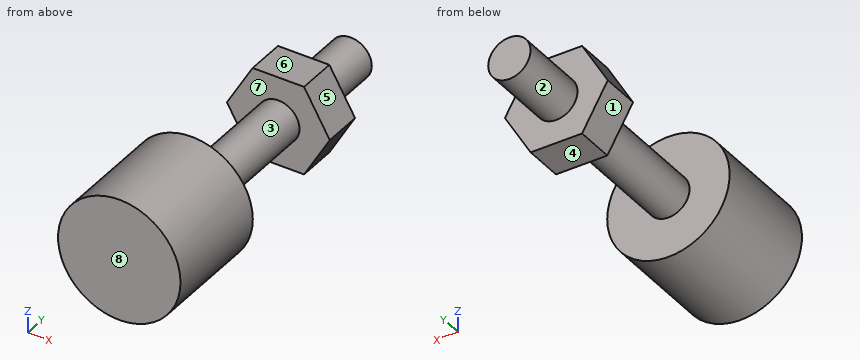
from build123d import *

# Parameters (mm, degrees)
F0_R     = 5.5
F0_R_2   = 1.9
F1_DEPTH = 10
F2_DEPTH = 22
F4_START = -6.5
F4_DEPTH = 3.5


with BuildPart() as f1:
    # F0 (on Front) → F1 (new body)
    with BuildSketch(Plane.XZ):
        Circle(F0_R)
        Circle(F0_R_2, mode=Mode.SUBTRACT)
        Circle(F0_R_2)
    extrude(amount=F1_DEPTH)

    # F0 (on Front) → F2 (join)
    with BuildSketch(Plane.XZ):
        Circle(F0_R_2)
    extrude(amount=-F2_DEPTH)

    # F3 (on face) → F4 (join)
    with BuildSketch(Plane(origin=(0, 22, 0), x_dir=(-1, 0, 0), z_dir=(0, 1, 0)).offset(F4_START)):
        Polygon((2.3094010768, 4), (-2.3094010768, 4), (-4.6188021535, 0), (-2.3094010768, -4), (2.3094010768, -4), (4.6188021535, 0), align=None)
    extrude(amount=-F4_DEPTH)


solid = f1.part
Build history of the part. All positions in model axes, mm. Face numbers are marked on the shaded views. A direction names the side the tool comes from. Give positions to 0.01 mm unless a question says otherwise; leave off trailing zeros. Order: outer loops, then holes, each group sorted by start corner. A loop starts at its lowest first (then second) coordinate and runs counter-clockwise, first axis right, second up. Notation, with made-up numbers: M 22.5,-35 L 57.5,-35 A29 cw 57.5,-6 Z; hole C 0.5,48 d8. An arc over 180 degrees is marked long. Use one line per item in the form item = value.
1) Saw through at C-C (y = -4). Give the cut face in (x, z), plus the area to 3 significant figures.
Calculated:
outline = C 0,0 d11
area = 95.0 mm2
2) Saw through at D-D (y = 16). Give the cut face in (x, z), plus the area to 3 significant figures.
Calculated:
outline = C 0,0 d3.8
area = 11.3 mm2
3) Saw through at A-A (x = 0). Give the cut face in (y, z), plus the area to 3 significant figures.
Calculated:
outline = M -10,-5.5 L 0,-5.5 L 0,-1.9 L 12,-1.9 L 12,-4 L 15.5,-4 L 15.5,-1.9 L 22,-1.9 L 22,1.9 L 15.5,1.9 L 15.5,4 L 12,4 L 12,1.9 L 0,1.9 L 0,5.5 L -10,5.5 Z
area = 208 mm2
4) Tool access for the marked faces 1, 2, 3, 4 and 5: list every direction of +Z, -Z, +X, -X, +Y, -Y with a clear straight run to the whole face (end or side of a thin tool).
Calculated:
face_1 = -Z, -X, +Y
face_2 = +Y
face_3 = none
face_4 = -Z, +X, -X, +Y
face_5 = +Z, +X, +Y
5) Saw through at B-B (z = 1). Give the cut face in (x, y).
Calculated:
outline = M -5.41,-10 L 5.41,-10 L 5.41,0 L 1.62,0 L 1.62,12 L 4.04,12 L 4.04,15.5 L 1.62,15.5 L 1.62,22 L -1.62,22 L -1.62,15.5 L -4.04,15.5 L -4.04,12 L -1.62,12 L -1.62,0 L -5.41,0 Z
6) Probe probe 1 along Y at (x, z) = (-3, -1.75); probe 2 along Y at (x, z) = (-5, -1.25); probe 3 along X at (y, z) = (16.5, -0.5). List the from-to ranges inside material, lowest first.
Calculated:
probe_1 = -10 to 0, 12 to 15.5
probe_2 = -10 to 0
probe_3 = -1.83 to 1.83
7) Two-plate mould, pull along Y, no slides. Class the marked faces 6, 7 and 8: released by +Y, released by -Y, zero draft, split by the parting line, or undercut.
Calculated:
face_6 = zero draft
face_7 = undercut
face_8 = released by -Y
8) Drop flat-ended pins along their axis: pin 1 (4 mm diameter, centred on x = 0, y = 14.5, fed in from -Z); pin 2 (4 mm diameter, centred on x = 2, z = 3.5, fed in from +Y); pin 3 (6 mm diameter, centred on y = -6, z = 3.5, fed in from -X). Give the stop position or say it passes through.
Calculated:
pin_1 = -4
pin_2 = 15.5
pin_3 = -5.48
